```python
from build123d import *

# Parameters (mm, degrees)
BOSS_EXTRUDE3_OUTLINE_W = 330.2
BOSS_EXTRUDE3_OUTLINE_H = 190.5
BOSS_EXTRUDE3_DEPTH     = 3
CUT_EXTRUDE2_DEPTH      = 554.733952504


# Read off the part's stored shape, not the designer's step: Boss-Extrude3
with BuildPart() as part:
    # Boss-Extrude3 outline → Boss-Extrude3 (new body)
    with BuildSketch(Plane.XY):
        with Locations((-165.1, -349.25)):
            Rectangle(BOSS_EXTRUDE3_OUTLINE_W, BOSS_EXTRUDE3_OUTLINE_H)
        with BuildLine():
            add(Edge.make_bspline(
                [(-278.621518652, -381.53819229), (-278.370340025, -381.675788485), (-277.859461829, -381.935426093), (-276.719402462, -382.422402226), (-274.453837446, -383.121197535), (-270.353871795, -383.430649395), (-265.517981506, -381.766237097), (-262.122707267, -378.912933368), (-260.111865445, -376.132298445), (-258.851133292, -372.940751822), (-258.274482706, -368.543399957), (-259.475297643, -363.572067472), (-261.943328375, -360.2835567), (-263.751900196, -358.750531033), (-264.776043253, -358.051952395), (-265.516797717, -357.615831636), (-266.283115012, -357.226375224), (-267.423174378, -356.739399091), (-269.688739395, -356.040603782), (-273.788705045, -355.731151923), (-278.624595335, -357.395564221), (-282.019869573, -360.248867949), (-284.030711396, -363.029502872), (-285.291443548, -366.221049495), (-285.868094135, -370.61840136), (-284.667279197, -375.589733845), (-282.199248466, -378.878244617), (-280.390676644, -380.411270284), (-279.366533588, -381.109848922), (-278.872697278, -381.400596095), (-278.621518652, -381.53819229)],
                knots=[0, 0, 0, 0, 0.015625, 0.03125, 0.0625, 0.125, 0.1875, 0.21875, 0.25, 0.28125, 0.3125, 0.375, 0.4375, 0.46875, 0.484375, 0.5, 0.515625, 0.53125, 0.5625, 0.625, 0.6875, 0.71875, 0.75, 0.78125, 0.8125, 0.875, 0.9375, 0.96875, 0.984375, 1, 1, 1, 1], degree=3))
        make_face(mode=Mode.SUBTRACT)
        with BuildLine():
            add(Edge.make_bspline(
                [(-158.330065967, -356.075599307), (-158.327001416, -356.373395786), (-158.290080957, -356.968671877), (-158.067598918, -358.246608867), (-157.224453748, -360.63292192), (-154.882508758, -363.615638807), (-150.614101822, -366.327010398), (-146.438166973, -368.010630749), (-141.434805852, -369.121724295), (-135.953318408, -369.477027412), (-130.480303716, -369.0089942), (-125.500867751, -367.795170138), (-121.360465048, -366.025968397), (-117.148760273, -363.227330056), (-114.868693567, -360.19704918), (-114.074835681, -357.79389013), (-113.878699845, -356.511645246), (-113.84170646, -355.617780511), (-113.897087149, -354.724866375), (-114.119569188, -353.446929384), (-114.962714357, -351.060616332), (-117.304659348, -348.077899444), (-121.573066284, -345.366527853), (-125.749001132, -343.682907503), (-130.752362254, -342.571813956), (-136.233849698, -342.216510839), (-141.70686439, -342.684544051), (-146.686300354, -343.898368114), (-150.826703058, -345.667569854), (-155.038407833, -348.466208196), (-157.318474538, -351.496489072), (-158.112332425, -353.899648121), (-158.30846826, -355.181893006), (-158.333130517, -355.777802829), (-158.330065967, -356.075599307)],
                knots=[0, 0, 0, 0, 0.015625, 0.03125, 0.0625, 0.125, 0.15625, 0.1875, 0.21875, 0.25, 0.28125, 0.3125, 0.34375, 0.375, 0.4375, 0.46875, 0.484375, 0.5, 0.515625, 0.53125, 0.5625, 0.625, 0.65625, 0.6875, 0.71875, 0.75, 0.78125, 0.8125, 0.84375, 0.875, 0.9375, 0.96875, 0.984375, 1, 1, 1, 1], degree=3))
        make_face(mode=Mode.SUBTRACT)
        with BuildLine():
            add(Edge.make_bspline(
                [(-33.964165547, -331.962198832), (-34.243868077, -332.023492326), (-34.799490244, -332.1633419), (-35.978750805, -332.544818645), (-38.145753578, -333.504844289), (-41.440772349, -335.959441018), (-43.995962688, -340.379536121), (-44.684039348, -344.749082337), (-44.375298942, -348.156558861), (-43.230759499, -351.380879931), (-40.778421797, -355.062241557), (-36.608937685, -358.008703948), (-32.589384281, -358.86039887), (-30.219493581, -358.826218077), (-28.988771838, -358.679575761), (-28.143989915, -358.521589154), (-27.310556664, -358.311814794), (-26.131296103, -357.930338049), (-23.96429333, -356.970312405), (-20.669274558, -354.515715676), (-18.11408422, -350.095620573), (-17.42600756, -345.726074356), (-17.734747965, -342.318597833), (-18.879287408, -339.094276763), (-21.331625111, -335.412915137), (-25.501109223, -332.466452745), (-29.520662627, -331.614757823), (-31.890553327, -331.648938617), (-33.121275069, -331.795580933), (-33.684463018, -331.900905337), (-33.964165547, -331.962198832)],
                knots=[0, 0, 0, 0, 0.015625, 0.03125, 0.0625, 0.125, 0.1875, 0.21875, 0.25, 0.28125, 0.3125, 0.375, 0.4375, 0.46875, 0.484375, 0.5, 0.515625, 0.53125, 0.5625, 0.625, 0.6875, 0.71875, 0.75, 0.78125, 0.8125, 0.875, 0.9375, 0.96875, 0.984375, 1, 1, 1, 1], degree=3))
        make_face(mode=Mode.SUBTRACT)
    extrude(amount=BOSS_EXTRUDE3_DEPTH)

    # Sketch9 → Cut-Extrude2 (cut, through all)
    with BuildSketch(Plane(origin=(0, 0, 0), x_dir=(-1, 0, 0), z_dir=(0, 0, -1))):
        with BuildLine():
            Line((0, -444.5), (330.2, -444.5))
            Line((330.2, -444.5), (330.2, -254))
            Line((330.2, -254), (271.955362236, -254))
            Line((271.955362236, -254), (271.955362236, -355.976421692))
            add(Edge.make_bspline(
                [(271.955362236, -355.976421692), (272.59093246, -355.976421692), (274.983557944, -356.142395301), (278.624595335, -357.395564221), (282.019869573, -360.248867949), (284.030711396, -363.029502872), (285.291443548, -366.221049495), (285.868094135, -370.61840136), (284.667279197, -375.589733845), (282.199248466, -378.878244617), (280.390676644, -380.411270284), (279.366533588, -381.109848922), (278.872697278, -381.400596095), (278.621518652, -381.53819229)],
                knots=[0.601106286, 0.601106286, 0.601106286, 0.601106286, 0.625, 0.6875, 0.71875, 0.75, 0.78125, 0.8125, 0.875, 0.9375, 0.96875, 0.984375, 1, 1, 1, 1], degree=3))
            add(Edge.make_bspline(
                [(278.621518652, -381.53819229), (278.370340025, -381.675788485), (277.859461829, -381.935426093), (276.719402462, -382.422402226), (274.88887928, -382.98701238), (273.070063108, -383.202935147), (271.955362236, -383.183342538)],
                knots=[0, 0, 0, 0, 0.015625, 0.03125, 0.0625, 0.103997424, 0.103997424, 0.103997424, 0.103997424], degree=3))
            Line((271.955362236, -383.183342538), (271.955362236, -389.89))
            Line((271.955362236, -389.89), (227.505362236, -389.89))
            Line((227.505362236, -389.89), (227.505362236, -326.39))
            Line((227.505362236, -326.39), (136.330752091, -326.39))
            Line((136.330752091, -326.39), (136.330752091, -342.354877875))
            add(Edge.make_bspline(
                [(136.330752091, -342.354877875), (138.123654962, -342.378162739), (141.736657922, -342.691806742), (146.686300354, -343.898368114), (150.826703058, -345.667569854), (155.038407833, -348.466208196), (157.318474538, -351.496489072), (158.112332425, -353.899648121), (158.30846826, -355.181893006), (158.333130517, -355.777802829), (158.330065967, -356.075599307)],
                knots=[0.750560936, 0.750560936, 0.750560936, 0.750560936, 0.78125, 0.8125, 0.84375, 0.875, 0.9375, 0.96875, 0.984375, 1, 1, 1, 1], degree=3))
            add(Edge.make_bspline(
                [(158.330065967, -356.075599307), (158.327001416, -356.373395786), (158.290080957, -356.968671877), (158.067598918, -358.246608867), (157.224453748, -360.63292192), (154.882508758, -363.615638807), (150.614101822, -366.327010398), (146.438166973, -368.010630749), (141.549303862, -369.096297788), (138.03098442, -369.341737675), (136.330752091, -369.341737675)],
                knots=[0, 0, 0, 0, 0.015625, 0.03125, 0.0625, 0.125, 0.15625, 0.1875, 0.21875, 0.247854605, 0.247854605, 0.247854605, 0.247854605], degree=3))
            Line((136.330752091, -369.341737675), (136.330752091, -377.19))
            Line((136.330752091, -377.19), (94.512592051, -377.19))
            Line((94.512592051, -377.19), (94.512592051, -326.39))
            Line((94.512592051, -326.39), (31.012592051, -326.39))
            Line((31.012592051, -326.39), (31.012592051, -331.651825694))
            add(Edge.make_bspline(
                [(31.012592051, -331.651825694), (31.419012916, -331.649248653), (32.140901517, -331.678767974), (33.121275069, -331.795580933), (33.684463018, -331.900905337), (33.964165547, -331.962198832)],
                knots=[0.950213485, 0.950213485, 0.950213485, 0.950213485, 0.96875, 0.984375, 1, 1, 1, 1], degree=3))
            add(Edge.make_bspline(
                [(33.964165547, -331.962198832), (34.243868077, -332.023492326), (34.799490244, -332.1633419), (35.978750805, -332.544818645), (38.145753578, -333.504844289), (41.440772349, -335.959441018), (43.995962688, -340.379536121), (44.684039348, -344.749082337), (44.375298942, -348.156558861), (43.230759499, -351.380879931), (40.778421797, -355.062241557), (36.608937685, -358.008703948), (33.032964836, -358.766409497), (31.318148935, -358.823600105), (31.012592051, -358.823600105)],
                knots=[0, 0, 0, 0, 0.015625, 0.03125, 0.0625, 0.125, 0.1875, 0.21875, 0.25, 0.28125, 0.3125, 0.375, 0.4375, 0.451506925, 0.451506925, 0.451506925, 0.451506925], degree=3))
            Line((31.012592051, -358.823600105), (31.012592051, -368.3))
            Line((31.012592051, -368.3), (0, -368.3))
            Line((0, -368.3), (0, -444.5))
        make_face()
    extrude(amount=-CUT_EXTRUDE2_DEPTH, mode=Mode.SUBTRACT)


solid = part.part
```
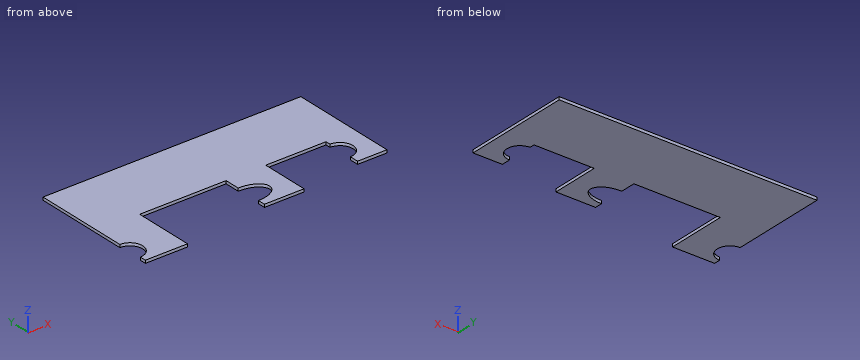
The listing builds one solid part. Answer for the finished solid, in the listing's coordinates (mm). Give positions to 0.01 mm unless a question says otherwise; leave off trailing zeros. Order: outer loops, then holes, each group sorted by start corner. A loop starts at its lowest first (then second) coordinate and runs counter-clockwise, first axis right, second up.
1) Given P1, Ø1.5, axis at x = -123, z = 1, coming from the -Y side; P2, Ø1.5, axis at y = -353.5, z = 1, coming from the +X side; P3, Ø0.9, axis at x = -63, z = 1, coming from the -Y side; P4, Ø1.5, axis at y = -374, z = 1.5, coming from the -X side, each flat-ended and moving along its own axis, determine where each tip first touches the part or whether it passes through.
Reported:
P1: stops at y = -377.19
P2: stops at x = 0
P3: stops at y = -326.39
P4: stops at x = -259.61
2) Find section A-A on x = -155. Write down the section's boundary in (y, z), then the cut area to 3 significant figures.
Reported:
outline: (-326.39, 0) - (-254, 0) - (-254, 3) - (-326.39, 3) - close
area: 217 mm2
3) Consider line 1 along X through (y, z) = (-369.5, 2.9); line 2 along Y through (x, z) = (-30, 2.2); line 3 along X through (y, z) = (-357, 1.6). Determine where each line is inside the solid, lowest interval first.
Reported:
line 1: x = -258.55 to -227.51, -136.33 to -94.51
line 2: y = -368.3 to -358.79, -331.7 to -254
line 3: x = -266.82 to -227.51, -113.96 to -94.51, -24.26 to 0
4) Find section B-B on y = -335. Give the number of separate pieces and of enclosed holes in the cut face, then the cut area to 3 significant figures.
Reported:
separate pieces: 3
enclosed holes: 0
area: 325 mm2
